```python
from build123d import *

# Parameters (mm, degrees)
SKETCH1_W             = 80
SKETCH1_H             = 64
SKETCH1_W_2           = 40.7
SKETCH1_H_2           = 40
BOSS_EXTRUDE1_DEPTH   = 15
SKETCH3_W             = 14
SKETCH3_H             = 11.1
SKETCH4_R             = 9.5
CUT_EXTRUDE2_DEPTH    = 81
SKETCH5_R             = 3
CUT_EXTRUDE3_DEPTH    = 65
SKETCH8_R             = 2.15
CUT_EXTRUDE6_DEPTH    = 16
FILLET1_R             = 20
CHAMFER1_SIZE         = 3
CHAMFER1_SIZE2        = 1.732050808
CHAMFER1_PART_2_SIZE  = 3
CHAMFER1_PART_2_SIZE2 = 1.732050808
SKETCH9_W             = 12
SKETCH9_H             = 3


with BuildPart() as part:
    # Sketch1 → Boss-Extrude1 (new body)
    with BuildSketch(Plane(origin=(0, 0, 0), x_dir=(1, 0, 0), z_dir=(0, 1, 0))):
        Rectangle(SKETCH1_W, SKETCH1_H)
        Rectangle(SKETCH1_W_2, SKETCH1_H_2, mode=Mode.SUBTRACT)
    extrude(amount=BOSS_EXTRUDE1_DEPTH)

    # Sketch3 → Cut-Revolve1 (revolve, cut)
    with BuildSketch(Plane(origin=(0, 15, 0), x_dir=(1, 0, 0), z_dir=(0, 1, 0))):
        with Locations((27.35, -5.55)):
            Rectangle(SKETCH3_W, SKETCH3_H)
        with Locations((-27.35, -5.55)):
            Rectangle(SKETCH3_W, SKETCH3_H)
    revolve(axis=Axis((20.35, 15, 0), (1, 0, 0)), mode=Mode.SUBTRACT)

    # Sketch4 → Cut-Extrude2 (cut, through all)
    with BuildSketch(Plane(origin=(40, 0, 0), x_dir=(0, 0, -1), z_dir=(1, 0, 0))):
        with Locations((0, 15)):
            Circle(SKETCH4_R)
    extrude(amount=-CUT_EXTRUDE2_DEPTH, mode=Mode.SUBTRACT)

    # Sketch5 → Cut-Extrude3 (cut, through all)
    with BuildSketch(Plane.XY.offset(32)):
        with Locations((0, 15)):
            Circle(SKETCH5_R)
    extrude(amount=-CUT_EXTRUDE3_DEPTH, mode=Mode.SUBTRACT)

    # Sketch8 → Cut-Extrude6 (cut, through all)
    with BuildSketch(Plane(origin=(0, 15, 0), x_dir=(1, 0, 0), z_dir=(0, 1, 0))):
        with Locations((24.5, 16.5)):
            Circle(SKETCH8_R)
        with Locations((24.5, -16.5)):
            Circle(SKETCH8_R)
        with Locations((-24.5, -16.5)):
            Circle(SKETCH8_R)
        with Locations((-24.5, 16.5)):
            Circle(SKETCH8_R)
        with Locations((9, -27)):
            Circle(SKETCH8_R)
        with Locations((-9, -27)):
            Circle(SKETCH8_R)
        with Locations((-9, 27)):
            Circle(SKETCH8_R)
        with Locations((9, 27)):
            Circle(SKETCH8_R)
        with Locations((-33, 16.5)):
            Circle(SKETCH8_R)
        with Locations((33, 16.5)):
            Circle(SKETCH8_R)
        with Locations((33, -16.5)):
            Circle(SKETCH8_R)
        with Locations((-33, -16.5)):
            Circle(SKETCH8_R)
    extrude(amount=-CUT_EXTRUDE6_DEPTH, mode=Mode.SUBTRACT)

    # Fillet1
    fillet1_edges = [part.edges().sort_by_distance(p)[0] for p in [
        (-40, 7.5, -32),
        (40, 7.5, -32),
        (40, 7.5, 32),
        (-40, 7.5, 32),
    ]]
    fillet(fillet1_edges, radius=FILLET1_R)

    # Chamfer1
    chamfer1_edges = [part.edges().sort_by_distance(p)[0] for p in [
        (20.35, 3.9, 0),
    ]]
    chamfer1_side = [part.faces().sort_by_distance(p)[0] for p in [
        (20.35, 0.427200187, 0),
    ]]
    chamfer(chamfer1_edges, length=CHAMFER1_SIZE, length2=CHAMFER1_SIZE2, reference=chamfer1_side[0])

    # Chamfer1 part 2
    chamfer1_part_2_edges = [part.edges().sort_by_distance(p)[0] for p in [
        (-20.35, 3.9, 0),
    ]]
    chamfer1_part_2_side = [part.faces().sort_by_distance(p)[0] for p in [
        (-20.35, 0.427200187, 0),
    ]]
    chamfer(chamfer1_part_2_edges, length=CHAMFER1_PART_2_SIZE, length2=CHAMFER1_PART_2_SIZE2, reference=chamfer1_part_2_side[0])

    # Sketch9 → Cut-Revolve2 (revolve, cut)
    with BuildSketch(Plane(origin=(0, 15, 0), x_dir=(1, 0, 0), z_dir=(0, 1, 0))):
        with Locations((-6, -21.5)):
            Rectangle(SKETCH9_W, SKETCH9_H)
        with Locations((-6, 21.5)):
            Rectangle(SKETCH9_W, SKETCH9_H)
    revolve(axis=Axis((0, 15, -29.871415895), (0, 0, 1)), mode=Mode.SUBTRACT)


solid = part.part
```
The model under review builds one solid part; all positions refer to its coordinate system, in mm. A direction names the side the tool comes from. Round coordinates to 2 decimals unless told otherwise and drop trailing zeros. Order: outer loops, then holes, each group sorted by start corner. A loop starts at its lowest first (then second) coordinate and runs counter-clockwise, first axis right, second up.
(1) Tool access review of faces 1 (the face through (0, 2, 20)), 2 (the face through (-37.135, 5.502, 0.209)), 3 (the face through (34.35, 5, 0)): name each direction out of +Z, -Z, +X, -X, +Y, -Y from which nothing blocks a thin tool from reaching the whole face with its end or side.
Working result:
face 1: +Y, -Y
face 2: +X, -X, +Y
face 3: +Y
(2) Take a section at D-D, the plane z = -16.5. State the section outline as (x, y) points, plus the area to 3 significant figures.
Working result:
outline: (-39.49, 0) - (-35.15, 0) - (-35.15, 15) - (-39.49, 15) - close; (-30.85, 0) - (-26.65, 0) - (-26.65, 15) - (-30.85, 15) - close; (-22.35, 0) - (-20.35, 0) - (-20.35, 15) - (-22.35, 15) - close; (20.35, 0) - (22.35, 0) - (22.35, 15) - (20.35, 15) - close; (26.65, 0) - (30.85, 0) - (30.85, 15) - (26.65, 15) - close; (35.15, 0) - (39.49, 0) - (39.49, 15) - (35.15, 15) - close
area: 316 mm2
(3) Mouldability with a two-part tool opening along Z and no side actions: class faces 4 (the face through (0, 3, -22)), 5 (the face through (-22, 15, 23)), 6 (the face through (-32.01, 7.6, -14.59)), 7 (the face through (33.986, 7.605, -26.297)) as released by +Z, released by -Z, zero draft, split by the parting line, or undercut.
Working result:
face 4: undercut
face 5: zero draft
face 6: undercut
face 7: released by -Z
(4) For P1, Ø5, axis at y = 10, z = 2.5, coming from the +X side; P2, Ø3, axis at x = 30.5, y = 3.5, coming from the +Z side; P3, Ø5, axis at y = 3.5, z = -18, coming from the -X side; P4, Ø2, axis at y = 10.5, z = 22, coming from the -X side, all flat-tipped, find the tip position at first contact; note any pin that passes through.
Working result:
P1: passes through
P2: stops at z = 29.86
P3: stops at x = -39.69
P4: stops at x = -37.86
(5) Take a section at B-B, the plane x = 0. State the section outline as (y, z) points, plus the area to 3 significant figures.
Working result:
outline: (0, -32) - (12, -32) - (12, -23) - (3, -23) - (3, -20) - (0, -20) - close; (0, 20) - (3, 20) - (3, 23) - (12, 23) - (12, 32) - (0, 32) - close
area: 234 mm2
(6) Take a section at A-A, the plane z = 0. State the section outline as (x, y) points, plus the area to 3 significant figures.
Working result:
outline: (-40, 0) - (-20.35, 0) - (-20.35, 0.9) - (-22.08, 3.9) - (-34.35, 3.9) - (-34.35, 5.5) - (-40, 5.5) - close; (20.35, 0) - (40, 0) - (40, 5.5) - (34.35, 5.5) - (34.35, 3.9) - (22.08, 3.9) - (20.35, 0.9) - close
area: 166 mm2
(7) Take a section at C-C, the plane x = 9. State the section outline as (y, z) points.
Working result:
outline: (0, -32) - (15, -32) - (15, -29.15) - (0, -29.15) - close; (0, -24.85) - (15, -24.85) - (15, -23) - (7.06, -23) - (7.06, -20) - (0, -20) - close; (0, 20) - (7.06, 20) - (7.06, 23) - (15, 23) - (15, 24.85) - (0, 24.85) - close; (0, 29.15) - (15, 29.15) - (15, 32) - (0, 32) - close
(8) Wall thickness on L1, parallel to Z at x = -9, y = 12; L2, parallel to Z at x = -4.5, y = 10.5; L3, parallel to X at y = 14, z = 11: over which ranges is each line inside the solid? List them lowest first.
Working result:
L1: z = -32 to -29.15, -24.85 to -23, 23 to 24.85, 29.15 to 32
L2: z = -32 to -23, 23 to 32
L3: x = -40 to -34.35, 34.35 to 40
